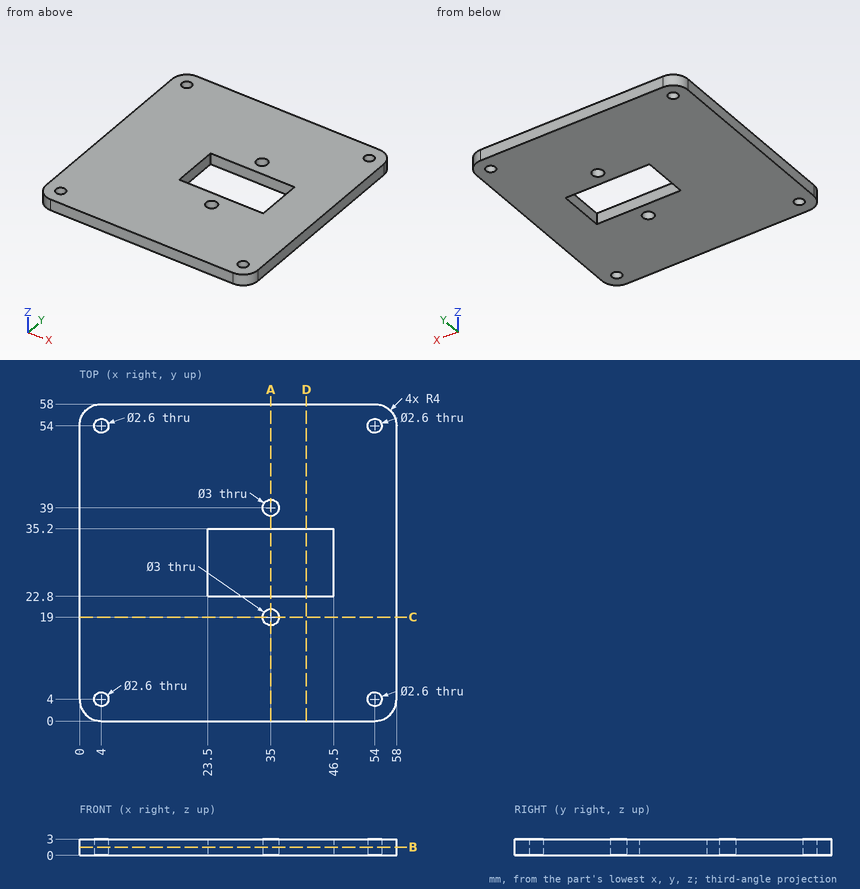
Can you work these out from the drawing? Everything is in mm from the part's minimum corner. Round coordinates to 2 decimals unless told otherwise and drop trailing zeros. Loops run counter-clockwise (first coordinate to the right, second up) from the corner with the lowest first, then second, coordinate; pieces in that order, holes last. Notation, with made-up numbers: (88.5, 59.25) - (147.5, 59.25) arc R26 ccw to (147.5, 96.25) - close; hole circle Ø4 at (2.5, -39). An arc over 180 degrees is marked (long way). One line per question, with ' | ' between items. Start each with the question number.
Q1. I want a section at B-B (z = 1.5). Write out the boundary of the cut face in (x, y).
Q2. I want a section at C-C (y = 19). Write out the boundary of the cut face in (x, z).
Q3. I want a section at D-D (x = 41.5). Write out the boundary of the cut face in (y, z).
Q4. Will this pin go through, and if not, where does the flat tip stop? pin 1 (2 mm diameter, centred on x = 54, y = 4, fed in from +Z).
Q5. I want a section at A-A (x = 35). Write out the boundary of the cut face in (y, z).
Q6. Please list where these lines run through material, in increasing order: line 1 (Y direction, x = 35, z = 1.1); line 2 (Y direction, x = 4, z = 2.1); line 3 (X direction, y = 24, z = 0.85). Write a range as [from, to].
Response values:
1) outline: (0, 4) arc R4 ccw to (4, 0) - (54, 0) arc R4 ccw to (58, 4) - (58, 54) arc R4 ccw to (54, 58) - (4, 58) arc R4 ccw to (0, 54) - close; hole circle Ø2.6 at (4, 4); hole circle Ø2.6 at (4, 54); hole (23.5, 22.8) - (46.5, 22.8) - (46.5, 35.2) - (23.5, 35.2) - close; hole circle Ø3 at (35, 19); hole circle Ø3 at (35, 39); hole circle Ø2.6 at (54, 4); hole circle Ø2.6 at (54, 54)
2) outline: (0, 0) - (33.5, 0) - (33.5, 3) - (0, 3) - close; (36.5, 0) - (58, 0) - (58, 3) - (36.5, 3) - close
3) outline: (0, 0) - (22.8, 0) - (22.8, 3) - (0, 3) - close; (35.2, 0) - (58, 0) - (58, 3) - (35.2, 3) - close
4) pin 1: passes through
5) outline: (0, 0) - (17.5, 0) - (17.5, 3) - (0, 3) - close; (20.5, 0) - (22.8, 0) - (22.8, 3) - (20.5, 3) - close; (35.2, 0) - (37.5, 0) - (37.5, 3) - (35.2, 3) - close; (40.5, 0) - (58, 0) - (58, 3) - (40.5, 3) - close
6) line 1: y = [0, 17.5], [20.5, 22.8], [35.2, 37.5], [40.5, 58] | line 2: y = [0, 2.7], [5.3, 52.7], [55.3, 58] | line 3: x = [0, 23.5], [46.5, 58]
